```python
from build123d import *

# Parameters (mm, degrees)
SKETCH_1_R      = 3.25
SKETCH_1_R_2    = 1.4
SKETCH_1_R_3    = 1
EXTRUDE_1_DEPTH = 3


with BuildPart() as part:
    # Эскиз1 → Бобышка-Вытянуть1 (new body)
    with BuildSketch(Plane.XY):
        with BuildLine():
            Line((1.6, -55.377499952), (8.119259302, -55.377499952))
            ThreePointArc((8.119259302, -55.377499952), (14.6, -53.377499952), (21.080740698, -55.377499952))
            Line((21.080740698, -55.377499952), (27.6, -55.377499952))
            ThreePointArc((27.6, -55.377499952), (31.135533906, -53.913033858), (32.6, -50.377499952))
            Line((32.6, -50.377499952), (32.6, -38.774674064))
            ThreePointArc((32.6, -38.774674064), (32.11800347, -35.002728245), (30.702989966, -31.473191066))
            Line((30.702989966, -31.473191066), (10.04562564, 5.597803631))
            ThreePointArc((10.04562564, 5.597803631), (-4.188430146, 10.710137857), (-11.17802813, -2.702163414))
            Line((-11.17802813, -2.702163414), (-3.679975539, -33.719326307))
            ThreePointArc((-3.679975539, -33.719326307), (-3.470240572, -34.885869352), (-3.4, -36.069033624))
            Line((-3.4, -36.069033624), (-3.4, -50.377499952))
            ThreePointArc((-3.4, -50.377499952), (-1.935533906, -53.913033858), (1.6, -55.377499952))
        make_face()
        Circle(SKETCH_1_R, mode=Mode.SUBTRACT)
        with Locations((-4.949747468, 4.949747468)):
            Circle(SKETCH_1_R_2, mode=Mode.SUBTRACT)
        with Locations((4.949747468, 4.949747468)):
            Circle(SKETCH_1_R_2, mode=Mode.SUBTRACT)
        with Locations((4.949747468, -4.949747468)):
            Circle(SKETCH_1_R_2, mode=Mode.SUBTRACT)
        with Locations((-4.949747468, -4.949747468)):
            Circle(SKETCH_1_R_2, mode=Mode.SUBTRACT)
        with Locations((7.1, -37.377499952)):
            Circle(SKETCH_1_R_3, mode=Mode.SUBTRACT)
        with Locations((22.1, -37.377499952)):
            Circle(SKETCH_1_R_3, mode=Mode.SUBTRACT)
        with Locations((7.1, -52.377499952)):
            Circle(SKETCH_1_R_3, mode=Mode.SUBTRACT)
        with Locations((22.1, -52.377499952)):
            Circle(SKETCH_1_R_3, mode=Mode.SUBTRACT)
        with Locations((14.6, -37.127499952)):
            Circle(SKETCH_1_R_3, mode=Mode.SUBTRACT)
        with Locations((21.6, -44.127499952)):
            Circle(SKETCH_1_R_3, mode=Mode.SUBTRACT)
        with Locations((7.6, -44.127499952)):
            Circle(SKETCH_1_R_3, mode=Mode.SUBTRACT)
    extrude(amount=-EXTRUDE_1_DEPTH)


solid = part.part
```
Read the model definition and answer for the solid it produces. Units are mm, in the model's axes. A direction names the side the tool comes from. Give positions to 0.01 mm unless a question says otherwise; leave off trailing zeros. Order: outer loops, then holes, each group sorted by start corner. A loop starts at its lowest first (then second) coordinate and runs counter-clockwise, first axis right, second up.
(1) Find section C-C (x = 0). Give the vertices of the cut face in (y, z).
(2) Given pin 1 (1.5 mm diameter, centred on y = -45.5, z = -1, fed in from -X); pin 2 (2.5 mm diameter, centred on x = 4.95, y = -4.95, fed in from +Z), each flat-ended and moving along its own axis, determine where each tip first touches the part or whether it passes through.
(3) For a pull along X with two mould halves and no side action, classify faces 1 (the cylindrical face through (6.97, -51.386, -1.479)), 2 (the flat face through (-7.481, -17.994, -1.479)), 3 (the flat face through (24, -55.377, -1)) as released by +X, released by -X, zero draft, split by the parting line, or undercut.
(4) For faces 4 (the cylindrical face through (21.97, -36.386, -1.479)), 5 (the flat face through (-3.4, -43, -1)), determine the directions among +Z, -Z, +X, -X, +Y, -Y from which every point of the face is accessible in a straight line to the end or side of a thin tool.
(5) Straight lines are drawn through the part: L1, parallel to X at y = -5, z = -1.75; L2, parallel to Y at x = 6, z = -2.55; L3, parallel to X at y = -38, z = -0.55. For each, find the intervals that lie inside material, in ascending order.
(6) Find section A-A (x = 14.6). Give the vertices of the cut face in (y, z), plus the area to 3 significant figures.
(7) Find section D-D (y = -30). Give the vertices of the cut face in (x, z), plus the area to 3 significant figures.
(8) Find section B-B (z = -2.4). Give the number of separate pieces and of enclosed holes in the cut face, plus the area to 3 significant figures.
Result sheet:
1. outline: (-55.11, -3) - (-3.25, -3) - (-3.25, 0) - (-55.11, 0) - close; (3.25, -3) - (11.5, -3) - (11.5, 0) - (3.25, 0) - close
2. pin 1: stops at x = -3.4
2. pin 2: passes through
3. face 1: undercut
3. face 2: released by -X
3. face 3: zero draft
4. face 4: +Z, -Z
4. face 5: +Z, -Z, -X, -Y
5. L1: x = -10.62 to -6.35, -3.55 to 3.55, 6.35 to 15.95
5. L2: y = -55.38 to -5.88, -4.02 to 4.02, 5.88 to 9.81
5. L3: x = -3.4 to 6.32, 7.88 to 14.11, 15.09 to 21.32, 22.88 to 32.58
6. outline: (-53.38, -3) - (-38.13, -3) - (-38.13, 0) - (-53.38, 0) - close; (-36.13, -3) - (-2.58, -3) - (-2.58, 0) - (-36.13, 0) - close
6. area: 146 mm2
7. outline: (-4.58, -3) - (29.88, -3) - (29.88, 0) - (-4.58, 0) - close
7. area: 103 mm2
8. separate pieces: 1
8. enclosed holes: 12
8. area: 1,900 mm2
